Build history of the part. All positions in model axes, mm. Round coordinates to 2 decimals unless told otherwise and drop trailing zeros. Use a Markdown table: item, result. Add a question column.
Item 1: Slice it at A-A, the plane y = 11.75. State how many separate pieces and enclosed holes the cut face has, plus the area to 3 significant figures.
Item 2: Pin check, flat tips, straight feed: pin 1 (5.5 mm diameter, centred on x = 10, z = 200, fed in from +Y); pin 2 (7.5 mm diameter, centred on x = 8.5, z = 920, fed in from +Y); pin 3 (5 mm diameter, centred on x = 8.5, z = 441, fed in from +Y). Stop position of each tip, or through.
Item 3: Probe L1, parallel to X at y = 12, z = 680; L2, parallel to X at y = 3.25, z = 980. List the from-to ranges inside material, lowest first.
Autodesk Inventor part; units mm, degrees
ref_plane "YZ Plane" through (0, 0, 0) normal (1, 0, 0) x (0, 1, 0)
ref_plane "XZ Plane" through (0, 0, 0) normal (0, 1, 0) x (-1, 0, 0)
ref_plane "XY Plane" through (0, 0, 0) normal (0, 0, 1) x (1, 0, 0)
sketch "Sketch1" plane through (0, 0, 0) normal (0, 0, 1) x (1, 0, 0)
  line L0 (0, 0) -> (20, 0)
  line L1 (20, 0) -> (20, 17.5)
  line L2 (20, 17.5) -> (0, 17.5)
  line L3 (0, 17.5) -> (0, 0)
  dimension "d0" = 20
  dimension "d1" = 17.5
extrude "Extrusion1" add sketch "Sketch1" along normal blind 1100
sketch "Sketch2" plane through (0, 17.5, 0) normal (0, 1, 0) x (1, 0, 0)
  circle A0 centre (10, -20) radius 3
  line L0 (20, 0) -> (0, 0)
  point P0 (10, 0)
  dimension "d4" = 6
  dimension "d5" = 20
extrude "Extrusion2" cut sketch "Sketch2" against normal up to surface (17.5 mm away)
sketch "Sketch3" plane through (0, 17.5, 0) normal (0, 1, 0) x (1, 0, 0)
  circle A0 centre (10, -20) radius 4.75
  circle A1 centre (10, -20) radius 3 construction
  point P0 (0, 0)
  dimension "d8" = 9.5
extrude "Extrusion3" cut sketch "Sketch3" against normal blind 8.5
pattern_linear "Rectangular Pattern1" count 18 spacing 60 along (0, 0, 1) of "Extrusion2", "Extrusion3"
properties part number "HGW20CC_Rack"
Check sheet entries:
| question | item | result |
|---|---|---|
| 1 | separate pieces | 1 |
| 1 | enclosed holes | 18 |
| 1 | area | 20,700 mm2 |
| 2 | pin 1 | through |
| 2 | pin 2 | y = 17.5 |
| 2 | pin 3 | y = 9 |
| 3 | L1 | 0 to 5.25, 14.75 to 20 |
| 3 | L2 | 0 to 7, 13 to 20 |
